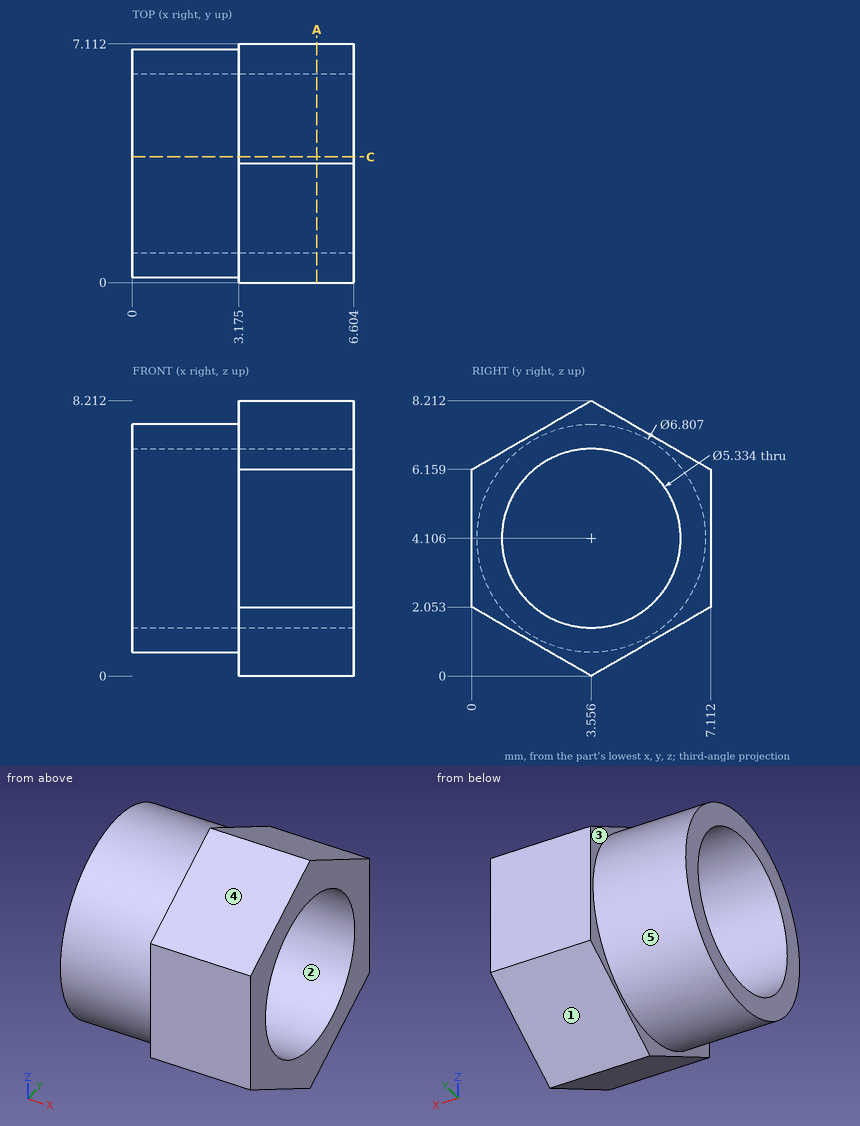
Answer from the drawing. Dimensions are ordinates in mm from the lowest x, y and z of the part. A direction names the side the tool comes from. Coordinates: 2 decimals unless noted, no trailing zeros. Loops run counter-clockwise (first coordinate to the right, second up) from the corner with the lowest first, then second, coordinate; pieces in that order, holes last.
Q1. The part is cut by section A-A on x = 5.5. Write down the section's boundary in (y, z).
Q2. The mould has two halves that part along Z. Classify the marked faces 1, 2 and 3: +Z half, -Z half, draft (parallel to the pull), parting line (faces both ways), or undercut.
Q3. Each of these flat-tipped pins is pushed along its axis until it touches: pin 1 Ø1.5 at (x, y) = (1, 3) entering from -Z; pin 2 Ø1 at (y, z) = (4.5, 4) entering from +X. Where does it stop, or does it pass through?
Q4. Consider probe 1 along Y at (x, z) = (4, 4); probe 2 along Z at (x, y) = (6, 5.75) (1 decimal); probe 3 along Z at (x, y) = (6.5, 4) (1 decimal). Determine where each line is inside the solid, lowest interval first.
Q5. Which of the six approach directions +Z, -Z, +X, -X, +Y, -Y give full straight-line access (tool end or side, diameter ignored) to the marked faces 4 and 5?
Q6. The part is cut by section C-C on y = 3.75. Write down the section's boundary in (x, z) (1 decimal).
Results below:
1. outline: (0, 2.05) - (3.56, 0) - (7.11, 2.05) - (7.11, 6.16) - (3.56, 8.21) - (0, 6.16) - close; hole circle Ø5.33 at (3.56, 4.11)
2. face 1: -Z half
2. face 2: undercut
2. face 3: draft
3. pin 1: stops at z = 0.7
3. pin 2: passes through
4. probe 1: y = 0 to 0.89, 6.22 to 7.11
4. probe 2: z = 1.3 to 2.6, 5.6 to 6.9
4. probe 3: z = 0.3 to 1.5, 6.7 to 8
5. face 4: +Z, +X, -X, -Y
5. face 5: -X
6. outline: (0, 0.7) - (3.2, 0.7) - (3.2, 0.1) - (6.6, 0.1) - (6.6, 1.4) - (0, 1.4) - close; (0, 6.8) - (6.6, 6.8) - (6.6, 8.1) - (3.2, 8.1) - (3.2, 7.5) - (0, 7.5) - close
